```python
from build123d import *

# Parameters (mm, degrees)
F4_W        = 51
F4_H        = 32
F5_DEPTH    = 60
F6_T1_DEPTH = 60
F7_R        = 4.42
F9_T1_DEPTH = 77.3960297945
F10_T       = -2
F11_R       = 11
F12_DEPTH   = 2
F13_R       = 51
F14_R       = 2


# Not quite as in the source:
# - a fillet or chamfer that OpenCascade refuses, or shapes differently, is made with other operations: its cross-section is extruded or revolved along the edge and cut away or added
# - two fillets or chamfers of one size are made in one step


with BuildPart() as f5:
    # F4 (on Top) → F5 (new body)
    with BuildSketch(Plane.XY):
        with BuildLine():
            Line((-25.5, 0), (-25.5, -2))
            Line((-25.5, -2), (25.5, -2))
            Line((25.5, -2), (25.5, 0))
            Line((25.5, 0), (4.7777200824, 0))
            ThreePointArc((4.7777200824, 0), (0, -1), (-4.7777200824, 0))
            Line((-4.7777200824, 0), (-25.5, 0))
        make_face()
        with Locations((0, -18)):
            Rectangle(F4_W, F4_H)
        with BuildLine():
            ThreePointArc((-8.9084552032, 18.8231877912), (-11.6364061524, 8.3597035712), (-4.7777200824, 0))
            Line((-4.7777200824, 0), (4.7777200824, 0))
            ThreePointArc((4.7777200824, 0), (11.6364061524, 8.3597035712), (8.9084552032, 18.8231877912))
            ThreePointArc((8.9084552032, 18.8231877912), (8.2131677669, 19.5429454632), (7.4599259019, 20.2018099548))
            ThreePointArc((7.4599259019, 20.2018099548), (0, 1), (-7.4599259019, 20.2018099548))
            ThreePointArc((-7.4599259019, 20.2018099548), (-8.2131677669, 19.5429454632), (-8.9084552032, 18.8231877912))
        make_face()
        with BuildLine():
            Line((4.7777200824, 0), (-4.7777200824, 0))
            ThreePointArc((-4.7777200824, 0), (0, -1), (4.7777200824, 0))
        make_face()
        with BuildLine():
            Line((-8.9084552032, 23.9303167421), (-8.9084552032, 18.8231877912))
            ThreePointArc((-8.9084552032, 18.8231877912), (-8.2131677669, 19.5429454632), (-7.4599259019, 20.2018099548))
            Line((-7.4599259019, 20.2018099548), (-8.9084552032, 23.9303167421))
        make_face()
        with BuildLine():
            ThreePointArc((7.4599259019, 20.2018099548), (8.2131677669, 19.5429454632), (8.9084552032, 18.8231877912))
            Line((8.9084552032, 18.8231877912), (8.9084552032, 23.9303167421))
            Line((8.9084552032, 23.9303167421), (7.4599259019, 20.2018099548))
        make_face()
    extrude(amount=F5_DEPTH)

    # F6: fillet of radius 110.5 on 2 edges, made by hand

    # F6_s2 → F6_t1 (join)
    with BuildSketch(Plane.XY):
        with BuildLine():
            ThreePointArc((-8.9084552032, 23.9303167421), (-10.0405186332, 19.1502401697), (-11.3839102474, 14.4252006335))
            ThreePointArc((-11.3839102474, 14.4252006335), (-10.3817434304, 16.7567821247), (-8.9084552032, 18.8231877912))
            Line((-8.9084552032, 18.8231877912), (-8.9084552032, 23.9303167421))
        make_face()
        with BuildLine():
            ThreePointArc((11.3839102474, 14.4252006335), (10.0405186332, 19.1502401697), (8.9084552032, 23.9303167421))
            Line((8.9084552032, 23.9303167421), (8.9084552032, 18.8231877912))
            ThreePointArc((8.9084552032, 18.8231877912), (10.3817434304, 16.7567821247), (11.3839102474, 14.4252006335))
        make_face()
    extrude(amount=F6_T1_DEPTH)

    # F7
    f7_edges = [f5.edges().sort_by_distance(p)[0] for p in [
        (-4.77772, 0, 30),
        (4.77772, 0, 30),
        (7.459926, 20.20181, 30),
        (-7.459926, 20.20181, 30),
    ]]
    fillet(f7_edges, radius=F7_R)

    # F9: fillet of radius 4.42 on 2 edges, made by hand

    # F9_s2 → F9_t1 (cut)
    with BuildSketch(Plane.XY.offset(-8.6980148973)):
        with BuildLine():
            ThreePointArc((9.6882803435, 20.5396314345), (9.2143493926, 21.7090785299), (8.4292935977, 22.6969572949))
            Line((8.4292935977, 22.6969572949), (8.9084552032, 23.9303167421))
            ThreePointArc((8.9084552032, 23.9303167421), (9.2850220453, 22.2319046987), (9.6882803435, 20.5396314345))
        make_face()
        with BuildLine():
            ThreePointArc((-9.6882803435, 20.5396314345), (-9.2143493926, 21.7090785299), (-8.4292935977, 22.6969572949))
            Line((-8.4292935977, 22.6969572949), (-8.9084552032, 23.9303167421))
            ThreePointArc((-8.9084552032, 23.9303167421), (-9.2850220453, 22.2319046987), (-9.6882803435, 20.5396314345))
        make_face()
    extrude(amount=F9_T1_DEPTH, mode=Mode.SUBTRACT)

    # F10
    f10_openings = [f5.faces().sort_by_distance(p)[0] for p in [
        (0, -15.707049, 60),
    ]]
    offset(amount=F10_T, openings=f10_openings)

    # F11 (on face) → F12 (cut)
    with BuildSketch(Plane(origin=(0, 0, 0), x_dir=(1, 0, 0), z_dir=(0, 0, -1))):
        with Locations((7.5, 20)):
            Circle(F11_R)
    extrude(amount=-F12_DEPTH, mode=Mode.SUBTRACT)

    # F13
    f13_edges = [f5.edges().sort_by_distance(p)[0] for p in [
        (-8.868399, 2.47639, 31),
        (8.868399, 2.47639, 31),
    ]]
    fillet(f13_edges, radius=F13_R)

    # F14
    f14_edges = [f5.edges().sort_by_distance(p)[0] for p in [
        (-25.5, 0, 30),
        (25.5, 0, 30),
        (23.5, -32, 31),
        (-23.5, -32, 31),
        (25.5, -34, 30),
        (-25.5, -34, 30),
        (23.5, -2, 31),
        (-23.5, -2, 31),
    ]]
    fillet(f14_edges, radius=F14_R)


solid = f5.part
```
Source: CAD feature listing. Evaluate the final solid. Frame: model axes, mm. A direction names the side the tool comes from. Coordinates: 2 decimals unless noted, no trailing zeros. Write each loop counter-clockwise with the first axis right and the second up, starting at its lowest first coordinate (ties: lowest second). Pieces come first, ordered by that corner, then holes. Notation, with made-up numbers: (14.5, 47) - (60.5, 47) arc R9 cw to (60.5, 53) - close; hole circle Ø4 at (75, -27). An arc over 180 degrees is marked (long way). Answer as a JSON object with one key per item and string values.
Q1. Draft query along X for faces 6 (the flat face through (0, -32, 31)), 7 (the cylindrical face through (11.33, 1.94, 30.42)), 8 (the cylindrical face through (-11.9, 10.32, 29.58)). Return one class per face: released by +X, released by -X, zero draft, split by the parting line, or undercut.
Ans:
{"face 6": "undercut", "face 7": "released by +X", "face 8": "released by -X"}
Q2. First-contact query: pin 1 Ø15.5 at (x, y) = (7, -12.5) entering from +Z; pin 2 Ø10 at (x, y) = (-17, 15.5) entering from +Z; pin 3 Ø7 at (x, z) = (17.5, 44) entering from +Y; pin 4 Ø7 at (x, z) = (-21, 22.5) entering from +Y. Flat tips, straight axial feed; report the tip coordinate or a pass-through.
Ans:
{"pin 1": "stops at z = 2", "pin 2": "passes through", "pin 3": "stops at y = 0.11", "pin 4": "stops at y = 0"}
Q3. Section query A-A, the plane y = 12.05. Output: boundary loops of the cut face in (x, z), plus the area to 3 significant figures.
Ans:
{"outline": "(-11.86, 0) - (-11.05, 0) - (-11.05, 60) - (-11.86, 60) - close; (11.05, 0) - (11.86, 0) - (11.86, 60) - (11.05, 60) - close", "area": "97.1 mm2"}
Q4. Material intervals for line 1 (Y direction, x = 15.5, z = 34); line 2 (X direction, y = -23.5, z = 53.5); line 3 (Y direction, x = 0, z = 39), sorted ascending. Write a range as [from, to].
Ans:
{"line 1": "y = [-34, -32], [-2, 0]", "line 2": "x = [-25.5, -23.5], [23.5, 25.5]", "line 3": "y = [-34, -32], [-1, 1]"}
Q5. Section query D-D, the plane y = -11.5. Output: boundary loops of the cut face in (x, z).
Ans:
{"outline": "(-25.5, 0) - (0.52, 0) - (0.52, 2) - (-23.5, 2) - (-23.5, 60) - (-25.5, 60) - close; (14.48, 0) - (25.5, 0) - (25.5, 60) - (23.5, 60) - (23.5, 2) - (14.48, 2) - close"}
Q6. Set-up query: faces 1 (the flat face through (25.5, -17, 30)), 2 (the cylindrical face through (-8.16, 20.57, 30.42)), 3 (the flat face through (19, 0, 30)), 4 (the cylindrical face through (22.93, -31.4, 30.59)), 5 (the cylindrical face through (-9.223, 21.694, 29.58)). Return all of +Z, -Z, +X, -X, +Y, -Y with unobstructed straight access to the full face (end or side cutting, diameter ignored); none if empty.
Ans:
{"face 1": "+Z, -Z, +X, +Y, -Y", "face 2": "+Z, -Z", "face 3": "+Z, -Z, +X, +Y", "face 4": "+Z", "face 5": "+Z, -Z, -X, +Y"}
Q7. Section query C-C, the plane x = -16. Output: boundary loops of the cut face in (y, z).
Ans:
{"outline": "(-34, 0) - (0, 0) - (0, 60) - (-2, 60) - (-2, 2) - (-32, 2) - (-32, 60) - (-34, 60) - close"}
Q8. Section query B-B, the plane x = 17.5. Output: boundary loops of the cut face in (y, z).
Ans:
{"outline": "(-34, 0) - (-24.58, 0) - (-24.58, 2) - (-32, 2) - (-32, 60) - (-34, 60) - close; (-15.42, 0) - (0, 0) - (0, 60) - (-2, 60) - (-2, 2) - (-15.42, 2) - close"}
